Design review of the part built by this model. Coordinates are the model's own, in mm. Face numbers are marked on the shaded views. A direction names the side the tool comes from. Round coordinates to 2 decimals unless told otherwise and drop trailing zeros. Write each loop counter-clockwise with the first axis right and the second up, starting at its lowest first coordinate (ties: lowest second). Pieces come first, ordered by that corner, then holes. Notation, with made-up numbers: (36.5, -35.75) -> (48.5, -35.75) arc R27 ccw to (48.5, -7.75) -> close; hole circle Ø4 at (68, 57). An arc over 180 degrees is marked (long way). One line per question, with ' | ' between items. Start each with the question number.
1) Insertion check: pin 1 Ø0.9 at (y, z) = (-13, 1.5) entering from +X; pin 2 Ø1.6 at (y, z) = (2, 1) entering from +X; pin 3 Ø0.9 at (y, z) = (8, 1) entering from -X. Each pin has a flat end and moves straight along its axis. Give the tip position at first contact, or say it passes through.
2) Mouldability with a two-part tool opening along X and no side actions: class the marked faces 1, 2, 3 and 4 as +X half, -X half, draft (parallel to the pull), parting line (faces both ways), or undercut.
3) Consider section B-B (y = 12). Give the boundary of the cut face in (x, z) (3 decimals), then the cut area to 3 significant figures.
4) For probe 1 along Y at (x, z) = (0.75, 2.6); probe 2 along X at (y, z) = (-8, 2.1); probe 3 along X at (y, z) = (6, 2.2), list the stretches that pass through material, from the lowest coordinate up.
5) Consider section A-A (z = 1.2). Give the boundary of the cut face in (x, y) (1 decimal).
6) Consider section C-C (y = -8). Give the boundary of the cut face in (x, z) (3 decimals).
7) Consider section D-D (x = -7.25). Give the boundary of the cut face in (y, z) (3 decimals).
8) For the marked faces 5, 6 and 7, list the 3-axis set-ups (+Z, -Z, +X, -X, +Y, -Y) from which the entire face can be reached by the end or side of a thin tool; tool diameter is ignored.
```python
from build123d import *

# Parameters (mm, degrees)
BOSS_EXTRUDE1_DEPTH = 3.125
FILLET1_R           = 7


with BuildPart() as part:
    # Sketch2 → Boss-Extrude1 (new body)
    with BuildSketch(Plane.XY):
        Polygon((0, 17), (5.5, 17), (5.5, 0.175), (8.68, 0.175), (8.68, 6.0875), (12.68, 6.0875), (12.68, -8.9125), (8.68, -8.9125), (8.68, -3), (5.5, -3), (5.5, -17), (0, -17), (0, 10.241210398), (1.59, 10.241210398), (1.59, 13.59), (0, 13.59), align=None)
    boss_extrude1 = extrude(amount=BOSS_EXTRUDE1_DEPTH)

    # Mirror1: Boss-Extrude1 across plane
    add(boss_extrude1.mirror(Plane(origin=(0, 10.241210398, 3.125), x_dir=(0, 0, 1), z_dir=(1, 0, 0))))

    # Fillet1
    # the kernel refuses this fillet: 7 mm, written as the material it takes off along each edge
    with BuildSketch(Plane(origin=(-12.68, -8.9125, -15.811388301), x_dir=(0, 1, 0), z_dir=(0, 0, 1)), Plane(origin=(12.68, 6.0875, -15.811388301), x_dir=(0, -1, 0), z_dir=(0, 0, 1))) as fillet1_piece_1:
        with BuildLine():
            CenterArc((6.32455532, -7), FILLET1_R, 90, 64.623066475)
            Line((0, -4), (-0.126491106, -3.94))
            ThreePointArc((-0.126491106, -3.94), (-0.14, -2), (-0.14, 0))
            Line((-0.14, 0), (0, 0.14))
            Line((0, 0.14), (6.32455532, 0.14))
            Line((6.32455532, 0.14), (6.32455532, 0))
        make_face()
    extrude(amount=34.747776602, mode=Mode.SUBTRACT)
    with BuildSketch(Plane(origin=(-12.68, 6.0875, -15.811388301), x_dir=(1, 0, 0), z_dir=(0, 0, 1)), Plane(origin=(12.68, -8.9125, -15.811388301), x_dir=(-1, 0, 0), z_dir=(0, 0, 1))) as fillet1_piece_2:
        with BuildLine():
            CenterArc((7, -6.32455532), FILLET1_R, 115.376933525, 64.623066475)
            Line((0, -6.32455532), (-0.14, -6.32455532))
            Line((-0.14, -6.32455532), (-0.14, 0))
            Line((-0.14, 0), (0, 0.14))
            ThreePointArc((0, 0.14), (2, 0.14), (3.94, 0.126491106))
            Line((3.94, 0.126491106), (4, 0))
        make_face()
    extrude(amount=34.747776602, mode=Mode.SUBTRACT)


solid = part.part
```
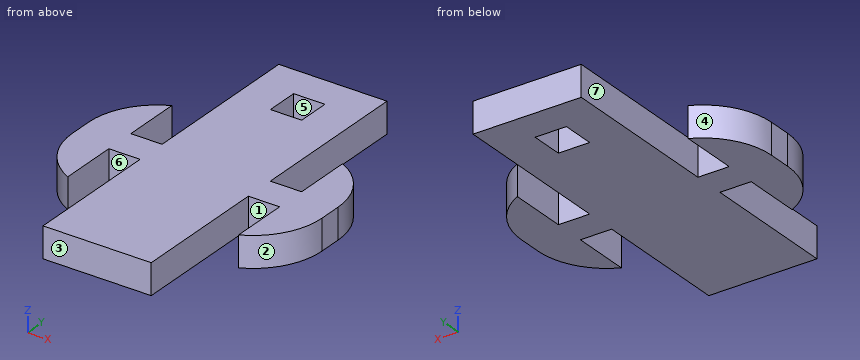
From the geometry:
1) pin 1: stops at x = 5.5 | pin 2: stops at x = 12.53 | pin 3: stops at x = -5.5
2) face 1: undercut | face 2: +X half | face 3: draft | face 4: -X half
3) outline: (-5.5, 0) -> (-1.59, 0) -> (-1.59, 3.125) -> (-5.5, 3.125) -> close; (1.59, 0) -> (5.5, 0) -> (5.5, 3.125) -> (1.59, 3.125) -> close | area: 24.4 mm2
4) probe 1: y = -17 to 10.24, 13.59 to 17 | probe 2: x = -10.12 to -8.68, -5.5 to 5.5, 8.68 to 10.12 | probe 3: x = -8.86 to -8.68, -5.5 to 5.5, 8.68 to 8.86
5) outline: (-12.7, -2.6) arc R7 ccw to (-8.7, -8.9) -> (-8.7, -3) -> (-5.5, -3) -> (-5.5, -17) -> (5.5, -17) -> (5.5, -3) -> (8.7, -3) -> (8.7, -8.9) arc R7 ccw to (12.7, -2.6) -> (12.7, -0.2) arc R7 ccw to (8.7, 6.1) -> (8.7, 0.2) -> (5.5, 0.2) -> (5.5, 17) -> (-5.5, 17) -> (-5.5, 0.2) -> (-8.7, 0.2) -> (-8.7, 6.1) arc R7 ccw to (-12.7, -0.2) -> close; hole (-1.6, 10.2) -> (1.6, 10.2) -> (1.6, 13.6) -> (-1.6, 13.6) -> close
6) outline: (-10.12, 0) -> (-8.68, 0) -> (-8.68, 3.125) -> (-10.12, 3.125) -> close; (-5.5, 0) -> (5.5, 0) -> (5.5, 3.125) -> (-5.5, 3.125) -> close; (8.68, 0) -> (10.12, 0) -> (10.12, 3.125) -> (8.68, 3.125) -> close
7) outline: (-3, 0) -> (0.175, 0) -> (0.175, 3.125) -> (-3, 3.125) -> close
8) face 5: +Z, -Z | face 6: +Z, -Z, -Y | face 7: +Z, -Z, +Y
